Could you check a few things on this drawing? It's one solid part, dimensions in mm from its lowest x, y, z. A direction names the side the tool comes from. Give positions to 0.01 mm unless a question says otherwise; leave off trailing zeros. Order: outer loops, then holes, each group sorted by start corner. A loop starts at its lowest first (then second) coordinate and runs counter-clockwise, first axis right, second up.
(1) Imagine slicing it at B-B, the plane x = 57. Write out the boundary of the cut face in (y, z).
(2) Imagine slicing it at A-A, the plane z = 7. Write out the boundary of the cut face in (x, y), then the cut area to 3 significant figures.
(3) If I drill on probe 1 along Z at (x, y) = (73, 1.1); probe 2 along X at (y, z) = (0.9, 20.75); probe 3 along Z at (x, y) = (11, 1.65), over which ranges is the centre line in solid material (lowest first)?
(4) Imagine slicing it at C-C, the plane x = 9. Write out the boundary of the cut face in (y, z), then the cut area to 3 significant figures.
(5) Imagine slicing it at D-D, the plane z = 20. Write out the boundary of the cut face in (x, y), then the cut area to 3 significant figures.
(6) On a 3-axis mill with a long thin cutter (end or side, diameter ignored), from which of +Z, -Z, +X, -X, +Y, -Y can I reach the whole of each face in a straight line? I mean the marked faces 1 and 2. Say none if no direction works.
(7) Will this pin go through, and if not, where does the flat tip stop? pin 1 (2 mm diameter, centred on x = 57.5, z = 19, fed in from -Y).
(8) If we mould it in two halves opening along Z, with no side actions, what happens to the marked faces 3, 4 and 5? For each: released by +Z, released by -Z, zero draft, split by the parting line, or undercut.
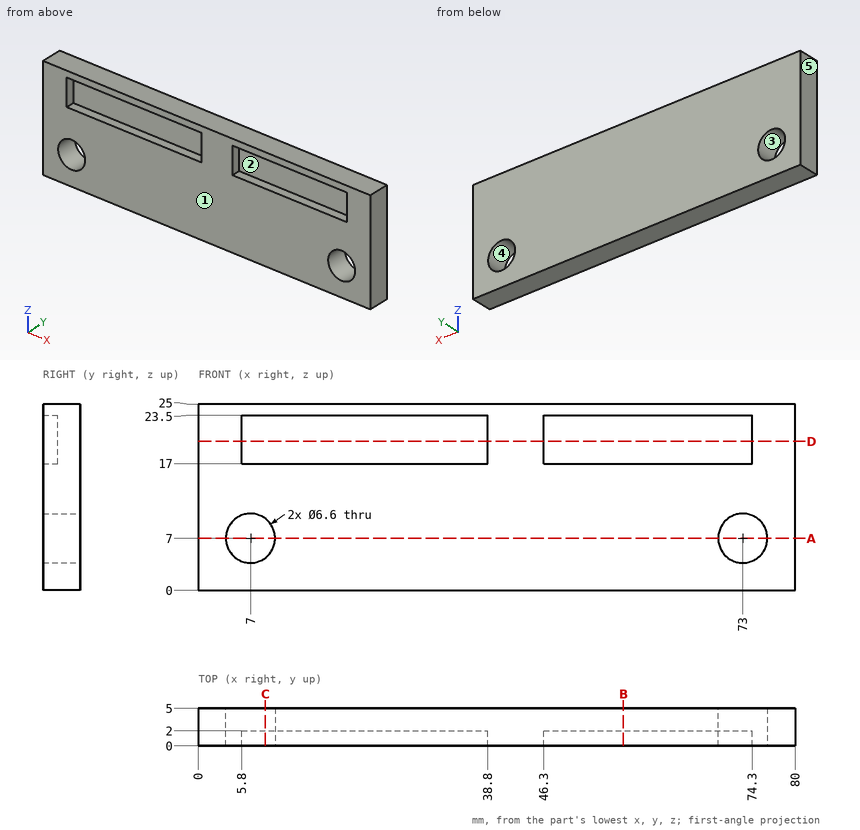
Answer block:
1. outline: (0, 0) - (5, 0) - (5, 25) - (0, 25) - (0, 23.5) - (2, 23.5) - (2, 17) - (0, 17) - close
2. outline: (0, 0) - (3.7, 0) - (3.7, 5) - (0, 5) - close; (10.3, 0) - (69.7, 0) - (69.7, 5) - (10.3, 5) - close; (76.3, 0) - (80, 0) - (80, 5) - (76.3, 5) - close
2. area: 334 mm2
3. probe 1: z = 0 to 3.7, 10.3 to 17, 23.5 to 25
3. probe 2: x = 0 to 5.8, 38.8 to 46.3, 74.3 to 80
3. probe 3: z = 0 to 17, 23.5 to 25
4. outline: (0, 0) - (5, 0) - (5, 4.38) - (0, 4.38) - close; (0, 9.62) - (5, 9.62) - (5, 25) - (0, 25) - (0, 23.5) - (2, 23.5) - (2, 17) - (0, 17) - close
4. area: 85.8 mm2
5. outline: (0, 0) - (5.8, 0) - (5.8, 2) - (38.8, 2) - (38.8, 0) - (46.3, 0) - (46.3, 2) - (74.3, 2) - (74.3, 0) - (80, 0) - (80, 5) - (0, 5) - close
5. area: 278 mm2
6. face 1: +Z, -Z, +X, -X, -Y
6. face 2: -Y
7. pin 1: stops at y = 2
8. face 3: undercut
8. face 4: undercut
8. face 5: zero draft
